Check sheet for the modelled part. Datum: model origin and axes. Units: mm. A direction names the side the tool comes from. Coordinates: 2 decimals unless noted, no trailing zeros. Loops run counter-clockwise (first coordinate to the right, second up) from the corner with the lowest first, then second, coordinate; pieces in that order, holes last. Notation, with made-up numbers: (68, 64.5) - (121, 64.5) arc R11 ccw to (121, 68.5) - close; hole circle Ø8 at (50.5, -3). An arc over 180 degrees is marked (long way). Answer as a JSON object with one key per item and string values. Group by question number.
from build123d import *

# Parameters (mm, degrees)
SKETCH1_R           = 10
BOSS_EXTRUDE1_DEPTH = 9
SKETCH2_R           = 14.5
BOSS_EXTRUDE2_DEPTH = 3
SKETCH3_R           = 14.5
SKETCH3_R_2         = 12
BOSS_EXTRUDE3_DEPTH = 10
SKETCH4_R           = 3
CUT_EXTRUDE1_DEPTH  = 13
BOSS_EXTRUDE4_REACH = 24
SKETCH5_R           = 1.5
CUT_EXTRUDE2_DEPTH  = 3.8
SKETCH7_R           = 22
SKETCH7_R_2         = 12
BOSS_EXTRUDE5_DEPTH = 6
SKETCH8_R           = 2.05
CUT_EXTRUDE3_DEPTH  = 5


with BuildPart() as part:
    # Sketch1 → Boss-Extrude1 (new body)
    with BuildSketch(Plane(origin=(0, 0, 0), x_dir=(1, 0, 0), z_dir=(0, 1, 0))):
        Circle(SKETCH1_R)
    extrude(amount=BOSS_EXTRUDE1_DEPTH)

    # Sketch2 → Boss-Extrude2 (add)
    with BuildSketch(Plane(origin=(0, 9, 0), x_dir=(1, 0, 0), z_dir=(0, 1, 0))):
        Circle(SKETCH2_R)
    extrude(amount=BOSS_EXTRUDE2_DEPTH)

    # Sketch3 → Boss-Extrude3 (add)
    with BuildSketch(Plane(origin=(0, 12, 0), x_dir=(1, 0, 0), z_dir=(0, 1, 0))):
        Circle(SKETCH3_R)
        Circle(SKETCH3_R_2, mode=Mode.SUBTRACT)
    extrude(amount=BOSS_EXTRUDE3_DEPTH)

    # Sketch4 → Cut-Extrude1 (cut, through all)
    with BuildSketch(Plane(origin=(0, 12, 0), x_dir=(1, 0, 0), z_dir=(0, 1, 0))):
        Circle(SKETCH4_R)
    extrude(amount=-CUT_EXTRUDE1_DEPTH, mode=Mode.SUBTRACT)

    # Sketch5 → Boss-Extrude4 (add, up to next)
    with BuildSketch(Plane.XZ, mode=Mode.PRIVATE) as boss_extrude4_sk1:
        with Locations((-13, 0)):
            Circle(SKETCH5_R)
    boss_extrude4_tool1 = extrude(boss_extrude4_sk1.sketch, amount=-BOSS_EXTRUDE4_REACH, mode=Mode.PRIVATE) - part.part
    add(boss_extrude4_tool1.solids().sort_by_distance((-13, 0, 0))[0])
    # Sketch5 → Boss-Extrude4 (add, up to next)
    with BuildSketch(Plane.XZ, mode=Mode.PRIVATE) as boss_extrude4_sk2:
        with BuildLine():
            ThreePointArc((-9.886859967, -1.5), (-10, 0), (-9.886859967, 1.5))
            Line((-9.886859967, 1.5), (-13, 1.5))
            ThreePointArc((-13, 1.5), (-11.939339828, 1.060660172), (-11.5, 0))
            ThreePointArc((-11.5, 0), (-11.939339828, -1.060660172), (-13, -1.5))
            Line((-13, -1.5), (-9.886859967, -1.5))
        make_face()
    boss_extrude4_tool2 = extrude(boss_extrude4_sk2.sketch, amount=-BOSS_EXTRUDE4_REACH, mode=Mode.PRIVATE) - part.part
    add(boss_extrude4_tool2.solids().sort_by_distance((-10.921971, 0, 0))[0])

    # Sketch6 → Cut-Extrude2 (cut)
    with BuildSketch(Plane(origin=(0, 3, 0), x_dir=(-1, 0, 0), z_dir=(0, -1, 0))):
        with BuildLine():
            Line((4, -2.309401077), (4, 2.309401077))
            Line((4, 2.309401077), (0, 4.618802154))
            Line((0, 4.618802154), (-4, 2.309401077))
            Line((-4, 2.309401077), (-4, -2.309401077))
            Line((-4, -2.309401077), (-4, -9.16515139))
            ThreePointArc((-4, -9.16515139), (0, -10), (4, -9.16515139))
            Line((4, -9.16515139), (4, -2.309401077))
        make_face()
    extrude(amount=-CUT_EXTRUDE2_DEPTH, mode=Mode.SUBTRACT)

    # Sketch7 → Boss-Extrude5 (add)
    with BuildSketch(Plane(origin=(0, 22, 0), x_dir=(1, 0, 0), z_dir=(0, 1, 0))):
        Circle(SKETCH7_R)
        Circle(SKETCH7_R_2, mode=Mode.SUBTRACT)
    extrude(amount=BOSS_EXTRUDE5_DEPTH)

    # Sketch8 → Cut-Extrude3 (cut)
    with BuildSketch(Plane(origin=(0, 28, 0), x_dir=(1, 0, 0), z_dir=(0, 1, 0))):
        with Locations((0, 17.5)):
            Circle(SKETCH8_R)
        with Locations((-7, -16)):
            Circle(SKETCH8_R)
        with Locations((7, -16)):
            Circle(SKETCH8_R)
    extrude(amount=-CUT_EXTRUDE3_DEPTH, mode=Mode.SUBTRACT)


solid = part.part
1. Gauge pin test, flat ends, axial feed: pin 1 (1.2 mm diameter, centred on x = -0.5, z = -16.5, fed in from +Y); pin 2 (8.5 mm diameter, centred on x = 6, z = 6, fed in from -Y); pin 3 (10 mm diameter, centred on x = 0.5, y = 20, fed in from -Z); pin 4 (2.5 mm diameter, centred on x = -0.5, z = 3, fed in from +Y). Record the tip position at first contact, or that the pin passes through.
2. Access from +Z, -Z, +X, -X, +Y, -Y to the whole of each face (thin tool, end or side, straight path). Record for faces 4 (the face through (3, 9, -10)), 5 (the face through (-11, 4, -1.5)), 6 (the face through (-2.028, 4.873, -3.448)), 7 (the face through (-8.627, 25.535, 17.247)), 8 (the face through (-14.5, 4.4, 0)).
3. Sectioned sample at C-C on x = 7. Record the cut outline in (y, z), plus the area to 3 significant figures.
4. Sectioned sample at A-A on y = 11.25. Record the cut outline in (x, z), plus the area to 3 significant figures.
5. Release check for a two-part mould opening along Y. For faces 1 (the face through (7, 23, 16)), 2 (the face through (-3, 9, 0)), 3 (the face through (1.97, 4.87, -3.48)) record: released by +Y, released by -Y, zero draft, split by the parting line, or undercut.
6. Material ranges on line 1 (Z direction, x = 0, y = 25.4); line 2 (X direction, y = 26.7, z = 16); line 3 (Z direction, x = 0, y = 21.25), recorded low to high.
7. Sectioned sample at D-D on y = 21.25. Record the cut outline in (x, z).
8. Sectioned sample at B-B on z = -16.5. Record the cut outline in (x, y), plus the area to 3 significant figures.
Answers follow:
{
 "1": {"pin 1": "stops at y = 23", "pin 2": "stops at y = 0", "pin 3": "stops at z = -22", "pin 4": "stops at y = 12"},
 "2": {"face 4": "-Y", "face 5": "-Z, -X, -Y", "face 6": "+Z", "face 7": "+Y", "face 8": "-X, -Y"},
 "3": {"outline": "(0, -7.14) - (9, -7.14) - (9, -12.7) - (22, -12.7) - (22, -20.86) - (28, -20.86) - (28, -9.75) - (12, -9.75) - (12, 9.75) - (28, 9.75) - (28, 13.95) - (23, 13.95) - (23, 18.05) - (28, 18.05) - (28, 20.86) - (22, 20.86) - (22, 12.7) - (9, 12.7) - (9, 7.14) - (0, 7.14) - close", "area": "377 mm^2"},
 "4": {"outline": "circle Ø29 at (0, 0); hole circle Ø6 at (0, 0)", "area": "632 mm^2"},
 "5": {"face 1": "released by +Y", "face 2": "zero draft", "face 3": "undercut"},
 "6": {"line 1": "z = -22 to -19.55, -15.45 to -12, 12 to 22", "line 2": "x = -15.1 to -9.05, -4.95 to 4.95, 9.05 to 15.1", "line 3": "z = -14.5 to -12, 12 to 14.5"},
 "7": {"outline": "circle Ø29 at (0, 0); hole circle Ø24 at (0, 0)"},
 "8": {"outline": "(-14.55, 22) - (14.55, 22) - (14.55, 28) - (1.79, 28) - (1.79, 23) - (-1.79, 23) - (-1.79, 28) - (-14.55, 28) - close", "area": "157 mm^2"}
}
